Input: part model. Units: mm. Frame: model coordinates. Face numbers are marked on the shaded views. Coordinates: 2 decimals unless noted, no trailing zeros. Write each loop counter-clockwise with the first axis right and the second up, starting at its lowest first coordinate (ties: lowest second). Pieces come first, ordered by that corner, then holes.
1) Line query: L1, parallel to Y at x = -11, z = 0; L2, parallel to Y at x = -19.5, z = 0; L3, parallel to X at y = -3.75, z = 2. Output: solid intervals per line, ascending.
2) Section query B-B (x = -15.25). Output: boundary loops of the cut face in (y, z) (1 decimal).
3) Draft query along Z for the marked faces 1, 2 and 3. Return one class per face: pulls with the +Z half, pulls with the -Z half, needs draft (parallel to the pull), parting line crosses it, or undercut.
4) Pin query (flat end, axial travel): pin 1 Ø1 at (x, z) = (-25, 5) entering from -Y; pin 2 Ø4 at (x, y) = (-20, -8.5) entering from -Z; pin 3 Ø1.5 at (x, z) = (-12.5, -5.5) entering from -Y. Return the tip coordinate at first contact, or that it passes through.
5) Section query A-A (x = -5.5). Output: boundary loops of the cut face in (y, z) (1 decimal), then the cut area to 3 significant figures.
from build123d import *

# Parameters (mm, degrees)
SKETCH3_R          = 7.9375
CUT_EXTRUDE1_DEPTH = 25.146
FILLET1_R          = 12.7


with BuildPart() as part:
    # Sketch2 → Revolve1 (revolve)
    with BuildSketch(Plane.XY, mode=Mode.PRIVATE) as revolve1_sk:
        Polygon((-27.809498475, 7.9375), (-27.809498475, 0), (-2.409498475, 0), (-2.409498475, 10.907816429), (-21.2812055, 10.186700377), align=None)
    revolve(revolve1_sk.sketch.rotate(Axis((-27.809498475, 0, 0), (1, 0, 0)), 90), axis=Axis((-27.809498475, 0, 0), (1, 0, 0)))

    # Sketch3 → Cut-Extrude1 (cut)
    with BuildSketch(Plane(origin=(-2.409498475, 0, 0), x_dir=(0, 0, -1), z_dir=(1, 0, 0))):
        Circle(SKETCH3_R)
    extrude(amount=-CUT_EXTRUDE1_DEPTH, mode=Mode.SUBTRACT)

    # Fillet1
    fillet1_edges = [part.edges().sort_by_distance(p)[0] for p in [
        (-21.2812055, 0, -10.186700377),
    ]]
    fillet(fillet1_edges, radius=FILLET1_R)


solid = part.part
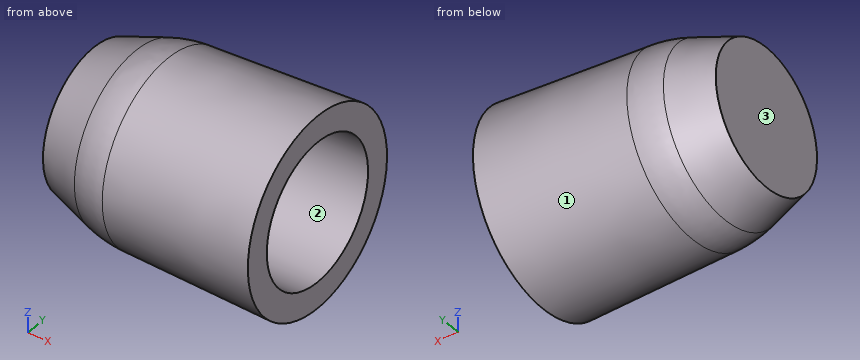
Answer:
1. L1: y = -10.58 to -7.94, 7.94 to 10.58
1. L2: y = -10.25 to -7.94, 7.94 to 10.25
1. L3: x = -27.81 to -27.56
2. outline: circle Ø20.8 at (0, 0); hole circle Ø15.9 at (0, 0)
3. face 1: parting line crosses it
3. face 2: undercut
3. face 3: needs draft
4. pin 1: stops at y = -7.75
4. pin 2: stops at z = -7.9
4. pin 3: stops at y = -9.39
5. outline: circle Ø21.6 at (0, 0); hole circle Ø15.9 at (0, 0)
5. area: 168 mm2
